CAD build for the part. Positions are in the model's coordinates, mm. A direction names the side the tool comes from. Coordinates: 2 decimals unless noted, no trailing zeros. Write each loop counter-clockwise with the first axis right and the second up, starting at its lowest first coordinate (ties: lowest second). Pieces come first, ordered by that corner, then holes. Notation, with made-up numbers: (54, -27.75) -> (87, -27.75) arc R23 cw to (87, -19.75) -> close; hole circle Ø8 at (48.5, -7.5). An arc over 180 degrees is marked (long way). Answer as CSV lines item,"result".
```python
from build123d import *

# Parameters (mm, degrees)
F0_R     = 17.75
F0_R_2   = 14.75
F1_DEPTH = 8
F3_R     = 7.5
F3_R_2   = 5
F4_DEPTH = 11
F5_W     = 2.4922459852
F5_H     = 8.3065871149
F6_DEPTH = 3
F8_COUNT = 8
F9_R     = 3
F10_R    = 2


with BuildPart() as f1:
    # F0 (on Top) → F1 (new body)
    with BuildSketch(Plane.XY):
        Circle(F0_R)
        Circle(F0_R_2, mode=Mode.SUBTRACT)
    extrude(amount=F1_DEPTH)



with BuildPart() as f4:
    # F3 (on offset) → F4 (new body)
    with BuildSketch(Plane.XY.offset(5)):
        Circle(F3_R)
        Circle(F3_R_2, mode=Mode.SUBTRACT)
    extrude(amount=F4_DEPTH)


with BuildPart() as f1_1:
    add(f1.part)

    add(f4.part)  # F6 merges F4
    # F5 (on offset) → F6 (join)
    with BuildSketch(Plane.XY.offset(5)):
        with Locations((0, 11.1227082089)):
            Rectangle(F5_W, F5_H)
    extrude(amount=F6_DEPTH)

    # F8: F1 ×8 about axis
    f8_axis = Axis((0, 0, 7.9989284277), (0, 0, -1))


with BuildPart() as f1_2:
    add(f1_1.part)
    for i in range(1, F8_COUNT):
        add(f1_1.part.rotate(f8_axis, i * 360 / F8_COUNT))

    # F9
    f9_edges = [f1_2.edges().sort_by_distance(p)[0] for p in [
        (7.473893, 0.625238, 8),
        (7.473893, -0.625238, 8),
        (5.303301, -5.303301, 8),
        (0, -7.5, 8),
        (-5.303301, -5.303301, 8),
        (-7.5, 0, 8),
        (-5.303301, 5.303301, 8),
        (0, 7.5, 8),
        (5.303301, 5.303301, 8),
        (14.736811, 0.623619, 5),
        (10.429825, 10.429825, 5),
        (0, 14.75, 5),
        (-10.429825, 10.429825, 5),
        (-14.75, 0, 5),
        (-10.429825, -10.429825, 5),
        (0, -14.75, 5),
        (10.429825, -10.429825, 5),
        (14.736811, -0.623619, 5),
    ]]
    fillet(f9_edges, radius=F9_R)

    # F10
    f10_edges = [f1_2.edges().sort_by_distance(p)[0] for p in [
        (-17.75, 0, 8),
        (-17.75, 0, 0),
        (-5, 0, 16),
    ]]
    fillet(f10_edges, radius=F10_R)


solid = f1_2.part
```
Item 1: Wall check: line 1 (Y direction, x = 0, z = 5.75); line 2 (X direction, y = -3.5, z = 7); line 3 (Z direction, x = 6, y = -4). Give the ranges that are in metal, low to high. Write a range as from..to.
Answer below:
line 1,"y = -17.75..-5, 5..17.75"
line 2,"x = -17.13..-14.33, -6.63..-3.57, 3.57..6.63, 14.33..17.13"
line 3,"z = 5..16"
Item 2: 3-axis set-ups, long thin cutter, end or side, ignore diameter. For faces 4 (the flat face through (11, -1.246, 6)), 5 (the flat face through (-2.7, 4.4, 5)), 6 (the cylindrical face through (6.93, -2.87, 11.65)): which of +Z, -Z, +X, -X, +Y, -Y reach the whole face in a straight line?
Answer below:
face 4,"+Z, -Z"
face 5,"-Z"
face 6,"+Z"
Item 3: Saw through at A-A on y = 0. Give the cut face in (x, z), and give its area (3 significant figures).
Answer below:
outline,"(-17.75, 2) arc R2 ccw to (-15.75, 0) -> (-14.75, 0) -> (-14.75, 2) arc R3 cw to (-11.75, 5) -> (-5, 5) -> (-5, 14) arc R2 ccw to (-7, 16) -> (-7.5, 16) -> (-7.5, 11) arc R3 cw to (-10.5, 8) -> (-15.75, 8) arc R2 ccw to (-17.75, 6) -> close; (5, 5) -> (11.75, 5) arc R3 cw to (14.75, 2) -> (14.75, 0) -> (15.75, 0) arc R2 ccw to (17.75, 2) -> (17.75, 6) arc R2 ccw to (15.75, 8) -> (10.5, 8) arc R3 cw to (7.5, 11) -> (7.5, 16) -> (7, 16) arc R2 ccw to (5, 14) -> close"
area,"149 mm2"
Item 4: Two-plate mould, pull along Y, no slides. Class faces 1 (the cylindrical face through (-1.08, -4.88, 9.44)), 2 (the cylindrical face through (-3.848, -17.328, 3.972)), 3 (the flat face through (7, 2, 16)): pulls with the +Y half, pulls with the -Y half, needs draft (parallel to the pull), parting line crosses it, or undercut.
Answer below:
face 1,"undercut"
face 2,"parting line crosses it"
face 3,"needs draft"
Item 5: Flat gauge pins, fed straight in: pin 1 (2 mm diameter, centred on x = -12, z = 5.5, fed in from +Y); pin 2 (5 mm diameter, centred on x = -1, y = -10.5, fed in from -Z); pin 3 (3.5 mm diameter, centred on y = -12.5, z = 8, fed in from -X); pin 4 (5 mm diameter, centred on y = -1.5, z = 3.5, fed in from -X). Where does each tip first touch, or does it go through?
Answer below:
pin 1,"stops at y = 13.93"
pin 2,"stops at z = 4.7"
pin 3,"stops at x = -13.54"
pin 4,"stops at x = -17.75"
Item 6: Saw through at D-D on y = 12.5. State how many separate pieces and enclosed holes the cut face has, and give its area (3 significant figures).
Answer below:
separate pieces,"3"
enclosed holes,"0"
area,"79.1 mm2"
